```python
from build123d import *

# Parameters (mm, degrees)
F3_DEPTH = 2.794
F4_R     = 1.898537
F5_DEPTH = 3.556


with BuildPart() as f2:
    # F1 (on Front) → F2 (revolve)
    with BuildSketch(Plane.XZ):
        with BuildLine():
            Line((0, 0), (0, -22.238212))
            ThreePointArc((0, -22.238212), (22.497638, -16.378549), (38.996805, 0))
            Line((38.996805, 0), (0, 0))
        make_face()
    revolve(axis=Axis((0, 0, -11.119106), (0, 0, -1)))

    # F0 (on Top) → F3 (join)
    with BuildSketch(Plane.XY):
        with BuildLine():
            Line((-38.1, 0), (38.1, 0))
            ThreePointArc((38.1, 0), (0, 38.1), (-38.1, 0))
        make_face()
        with BuildLine():
            ThreePointArc((-38.1, 0), (0, -38.1), (38.1, 0))
            Line((38.1, 0), (-38.1, 0))
        make_face()
    extrude(amount=F3_DEPTH)

    # F4 (on Top) → F5 (join, symmetric)
    with BuildSketch(Plane.XY):
        with Locations((-38.242929, 0)):
            Circle(F4_R)
        with Locations((0, -38.242929)):
            Circle(F4_R)
        with Locations((38.242929, 0)):
            Circle(F4_R)
        with Locations((0, 38.242929)):
            Circle(F4_R)
    extrude(amount=F5_DEPTH, both=True)


solid = f2.part
```
For this review, take the finished solid that the model builds, in its own axes (mm). A direction names the side the tool comes from. Round coordinates to 2 decimals unless told otherwise and drop trailing zeros. Answer as a JSON object with one key per item and string values.
1. For pin 1 Ø3 at (x, y) = (-0.5, -38) entering from -Z; pin 2 Ø3 at (y, z) = (-3.5, -13.5) entering from +X; pin 3 Ø23 at (x, y) = (-4, 15) entering from +Z, all flat-tipped, find the tip position at first contact; note any pin that passes through.
Response values:
{"pin 1": "stops at z = -3.83", "pin 2": "stops at x = 28.63", "pin 3": "stops at z = 2.79"}
2. Tool access review of faces 1 (the face through (38, 0, -3.556)), 2 (the face through (0, 38, -3.556)), 3 (the face through (-27.3, -27.3, 0)): name each direction out of +Z, -Z, +X, -X, +Y, -Y from which nothing blocks a thin tool from reaching the whole face with its end or side.
Response values:
{"face 1": "-Z, +X, +Y, -Y", "face 2": "-Z, +X, -X, +Y", "face 3": "+Z, -X, -Y"}
3. To check wall thickness, follow line 1 along Z through (x, y) = (-27.5, 11.5); line 2 along Z through (x, y) = (24, -12); line 3 along X through (y, z) = (20.5, -11.5). State the ranges of each line that lie inside material, in increasing order.
Response values:
{"line 1": "z = -11.17 to 2.79", "line 2": "z = -13.56 to 2.79", "line 3": "x = -21.11 to 21.11"}
